Geometry: see drawing. Coordinates: mm, zero at the bounding-box minimum. A direction names the side the tool comes from. Coordinates: 2 decimals unless noted, no trailing zeros. Order: outer loops, then holes, each group sorted by start corner. A loop starts at its lowest first (then second) coordinate and runs counter-clockwise, first axis right, second up.
Item 1: Reachability of the marked faces 5, 6 and 7 from +Z, -Z, +X, -X, +Y, -Y: full face, straight path, thin tool, end or side. Return the list, or none.
Item 2: Section D-D on y = 26.5. Return the cut outline in (x, z).
Item 3: Ray query, line 1 (X direction, y = 60, z = 35); line 2 (Z direction, x = 110.5, y = 41); line 3 (Z direction, x = 72, y = 32). Return the intervals inside material, ascending.
Item 4: Section C-C on x = 50.5. Return the cut outline in (y, z).
Item 5: Contact query for flat-ended pins moving along their axis: P1, Ø8, axis at y = 43, z = 5, coming from the +X side; P2, Ø6.5, axis at y = 26.5, z = 8, coming from the -X side; P3, Ø12, axis at x = 45.5, y = 27.5, coming from the +Z side. Output: stop coordinate, or through.
Item 6: Section B-B on z = 3.5. Return the cut outline in (x, y), then the cut area to 3 significant figures.
Item 7: Section A-A on y = 7. Return the cut outline in (x, z), then the cut area to 3 significant figures.
Item 8: Mould query, pull axis X, two halves, no side actions, for the marked faces 1, 2, 3 and 4. Classes: released by +X, released by -X, zero draft, split by the parting line, or undercut.
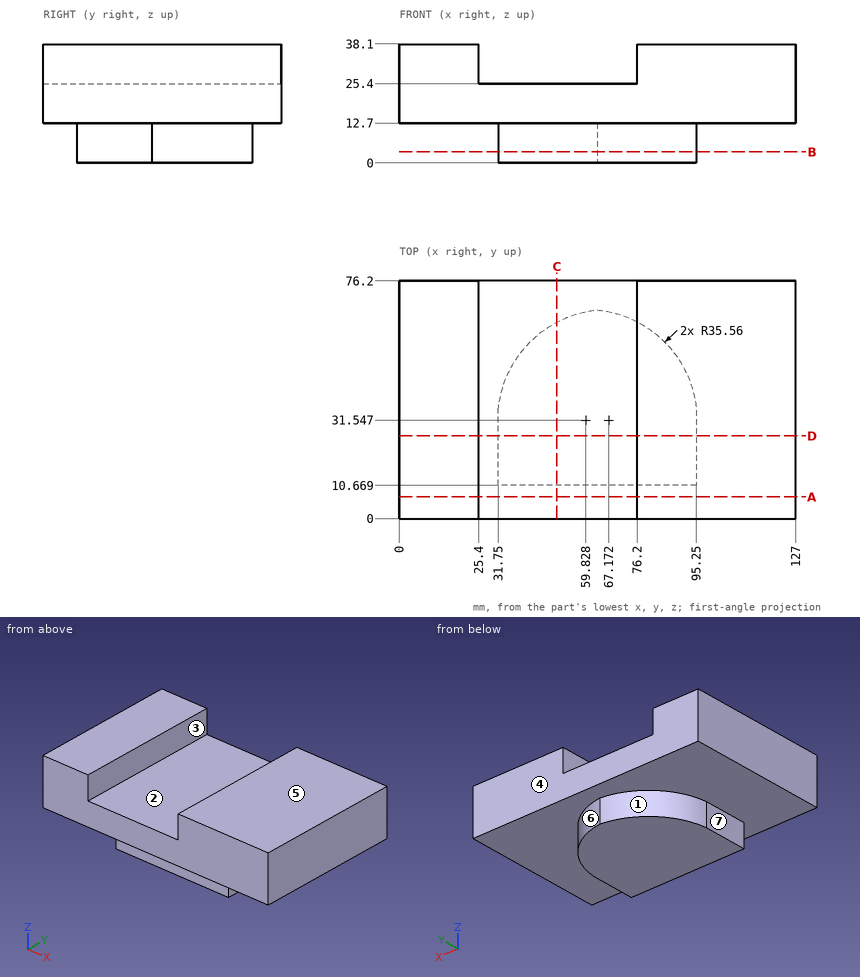
Answer list:
1. face 5: +Z, +X, -X, +Y, -Y
1. face 6: -Z, +X, +Y
1. face 7: -Z, -X, +Y, -Y
2. outline: (0, 12.7) - (31.75, 12.7) - (31.75, 0) - (95.25, 0) - (95.25, 12.7) - (127, 12.7) - (127, 38.1) - (76.2, 38.1) - (76.2, 25.4) - (25.4, 25.4) - (25.4, 38.1) - (0, 38.1) - close
3. line 1: x = 0 to 25.4, 76.2 to 127
3. line 2: z = 12.7 to 38.1
3. line 3: z = 0 to 25.4
4. outline: (0, 12.7) - (10.67, 12.7) - (10.67, 0) - (62.96, 0) - (62.96, 12.7) - (76.2, 12.7) - (76.2, 25.4) - (0, 25.4) - close
5. P1: stops at x = 94.6
5. P2: stops at x = 31.75
5. P3: stops at z = 25.4
6. outline: (31.75, 10.67) - (95.25, 10.67) - (95.25, 34.68) arc R35.56 ccw to (63.5, 66.92) arc R35.56 ccw to (31.75, 34.68) - close
6. area: 3,050 mm2
7. outline: (0, 12.7) - (127, 12.7) - (127, 38.1) - (76.2, 38.1) - (76.2, 25.4) - (25.4, 25.4) - (25.4, 38.1) - (0, 38.1) - close
7. area: 2,580 mm2
8. face 1: released by -X
8. face 2: undercut
8. face 3: undercut
8. face 4: zero draft
